Here's how the part is built. I have some questions about the finished solid (model axes, mm). Face numbers are marked on the shaded views. Give positions to 0.01 mm unless a question says otherwise; leave off trailing zeros. Order: outer loops, then holes, each group sorted by start corner. A loop starts at its lowest first (then second) coordinate and runs counter-clockwise, first axis right, second up.
from build123d import *

# Parameters (mm, degrees)
F0_W     = 40
F0_H     = 40
F0_R     = 1.75
F0_R_2   = 19
F1_DEPTH = 7
F2_R     = 1


with BuildPart() as f1:
    # F0 (on Front) → F1 (new body)
    with BuildSketch(Plane.XZ):
        Rectangle(F0_W, F0_H)
        with Locations((-16, -16)):
            Circle(F0_R, mode=Mode.SUBTRACT)
        with Locations((16, -16)):
            Circle(F0_R, mode=Mode.SUBTRACT)
        with Locations((-16, 16)):
            Circle(F0_R, mode=Mode.SUBTRACT)
        Circle(F0_R_2, mode=Mode.SUBTRACT)
        with Locations((16, 16)):
            Circle(F0_R, mode=Mode.SUBTRACT)
    extrude(amount=F1_DEPTH)

    # F2
    f2_edges = [f1.edges().sort_by_distance(p)[0] for p in [
        (20, -3.5, -20),
        (-20, -3.5, -20),
        (20, -3.5, 20),
        (-20, -3.5, 20),
    ]]
    fillet(f2_edges, radius=F2_R)


solid = f1.part
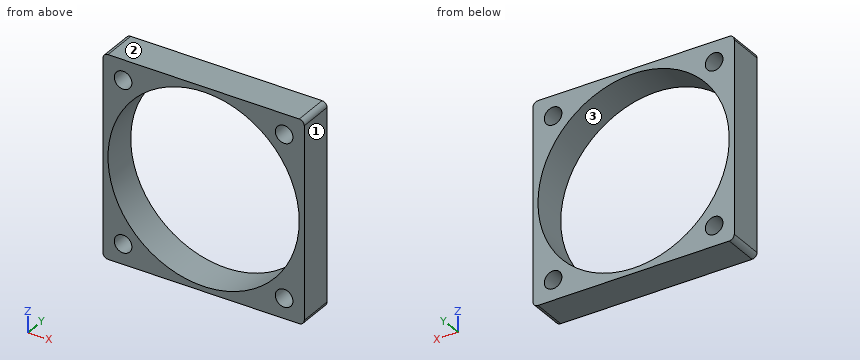
Q1. If we section it at C-C on y = -6: List the corners of the cut face in (x, z) for me, plus the area to 3 significant figures.
Filled sheet:
outline: (-20, -19) arc R1 ccw to (-19, -20) - (19, -20) arc R1 ccw to (20, -19) - (20, 19) arc R1 ccw to (19, 20) - (-19, 20) arc R1 ccw to (-20, 19) - close; hole circle Ø38 at (0, 0); hole circle Ø3.5 at (-16, -16); hole circle Ø3.5 at (-16, 16); hole circle Ø3.5 at (16, -16); hole circle Ø3.5 at (16, 16)
area: 427 mm2
Q2. If we section it at D-D on x = 16: List the corners of the cut face in (y, z) for me.
Filled sheet:
outline: (-7, -20) - (0, -20) - (0, -17.75) - (-7, -17.75) - close; (-7, -14.25) - (0, -14.25) - (0, -10.25) - (-7, -10.25) - close; (-7, 10.25) - (0, 10.25) - (0, 14.25) - (-7, 14.25) - close; (-7, 17.75) - (0, 17.75) - (0, 20) - (-7, 20) - close
Q3. If we section it at A-A on z = 0: List the corners of the cut face in (x, y) for me.
Filled sheet:
outline: (-20, -7) - (-19, -7) - (-19, 0) - (-20, 0) - close; (19, -7) - (20, -7) - (20, 0) - (19, 0) - close
Q4. Thinking about a two-plate mould opening in X: for the marked faces 1, 2 and 3, which applies, released by +X, released by -X, zero draft, split by the parting line, or undercut?
Filled sheet:
face 1: released by +X
face 2: zero draft
face 3: undercut
Q5. I need wall thicknesses on L1, parallel to X at y = -2, z = 17; L2, parallel to Z at x = 16, y = -5.5; L3, parallel to Z at x = 0, y = -4.75. Which ranges of each line are inside material? Lowest first, please.
Filled sheet:
L1: x = -20 to -17.44, -14.56 to -8.49, 8.49 to 14.56, 17.44 to 20
L2: z = -20 to -17.75, -14.25 to -10.25, 10.25 to 14.25, 17.75 to 20
L3: z = -20 to -19, 19 to 20
Q6. If we section it at B-B on x = 3: List the corners of the cut face in (y, z) for me.
Filled sheet:
outline: (-7, -20) - (0, -20) - (0, -18.76) - (-7, -18.76) - close; (-7, 18.76) - (0, 18.76) - (0, 20) - (-7, 20) - close
Q7. I'm going to push a flat-ended pin straight in: P1, Ø3, axis at x = -16, z = -16, coming from the -Y side. Where does the tip first touch, or does it pass through?
Filled sheet:
P1: passes through
